Autodesk Inventor part; units mm, degrees
ref_plane "YZ Plane" through (0, 0, 0) normal (1, 0, 0) x (0, 1, 0)
ref_plane "XZ Plane" through (0, 0, 0) normal (0, 1, 0) x (-1, 0, 0)
ref_plane "XY Plane" through (0, 0, 0) normal (0, 0, 1) x (1, 0, 0)
sketch "Sketch1" plane through (0, 0, 0) normal (0, 1, 0) x (-1, 0, 0)
  line L0 (9.5, 7.5) -> (-9.5, 7.5)
  line L1 (-9.5, 7.5) -> (-9.5, -7.5)
  line L2 (-9.5, -7.5) -> (9.5, -7.5)
  line L3 (9.5, -7.5) -> (9.5, 7.5)
  line L4 (9.5, 7.5) -> (-9.5, -7.5) construction
  line L5 (-9.5, 7.5) -> (9.5, -7.5) construction
  line L6 (7.5, 5.5) -> (-7.5, 5.5)
  line L7 (-7.5, 5.5) -> (-7.5, -5.5)
  line L8 (-7.5, -5.5) -> (7.5, -5.5)
  line L9 (7.5, -5.5) -> (7.5, 5.5)
  line L10 (7.5, 5.5) -> (-7.5, -5.5) construction
  line L11 (-7.5, 5.5) -> (7.5, -5.5) construction
  point P0 (0, 0)
  dimension "d0" = 19
  dimension "d1" = 15
  dimension "d2" = 2
  dimension "d3" = 2
extrude "Extrusion1" add sketch "Sketch1" along normal blind 115
sketch "Sketch3" plane through (0, 0, 0) normal (0, -1, 0) x (1, 0, 0)
  circle A0 centre (2.5, 11.5) radius 2.5
  circle A1 centre (2.5, -11.5) radius 2.5
  line L0 (-9.5, -7.5) -> (-9.5, 7.5)
  line L1 (-9.5, 7.5) -> (9.5, 7.5)
  line L2 (-2, 7.5) -> (7, 7.5)
  line L3 (7, 7.5) -> (7, 16.5)
  line L4 (7, 16.5) -> (-2, 16.5)
  line L5 (-2, 16.5) -> (-2, 7.5)
  line L6 (0, 0) -> (7.5, 0)
  line L7 (7.5, -5.5) -> (7.5, 5.5)
  circle A2 centre (2.5, -11.5) radius 2.5
  line L8 (-9.5, -7.5) -> (9.5, -7.5)
  line L9 (7, -7.5) -> (7, -16.5)
  line L10 (7, -16.5) -> (-2, -16.5)
  line L11 (-2, -16.5) -> (-2, -7.5)
  dimension "d13" = 5
  dimension "d14" = 5
  dimension "d15" = 23
  dimension "d16" = 11.5
  dimension "d17" = 12
  dimension "d18" = 12
  dimension "d19" = 9
  dimension "d20" = 9
  dimension "d21" = 4.5
extrude "Extrusion3" add sketch "Sketch3" against normal blind 3
fillet "Fillet2" radius 2 8 edges at (-2, 1.5, -7.5) (-2, 1.5, -16.5) (7, 1.5, -16.5) (7, 1.5, -7.5) (7, 1.5, 7.5) (7, 1.5, 16.5) (-2, 1.5, 16.5) (-2, 1.5, 7.5)
sketch "Sketch2" plane through (0, 0, 0) normal (0, -1, 0) x (1, 0, 0)
  circle A0 centre (-11.5, 0) radius 2.5
  circle A1 centre (11.5, 0) radius 2.5
  line L0 (-14.8361, 4.3238) -> (-8.1639, 4.3238)
  line L1 (-8.1639, 4.3238) -> (-8.1639, -4.3238)
  line L2 (-8.1639, -4.3238) -> (-14.8361, -4.3238)
  line L3 (-14.8361, -4.3238) -> (-14.8361, 4.3238)
  line L4 (-14.8361, 4.3238) -> (-8.1639, -4.3238) construction
  line L5 (-8.1639, 4.3238) -> (-14.8361, -4.3238) construction
  line L6 (0, 0) -> (0, 5.5)
  line L7 (7.5, 5.5) -> (-7.5, 5.5)
  line L8 (14.8361, 4.3238) -> (8.1639, 4.3238)
  line L9 (8.1639, 4.3238) -> (8.1639, -4.3238)
  line L10 (8.1639, -4.3238) -> (14.8361, -4.3238)
  line L11 (14.8361, -4.3238) -> (14.8361, 4.3238)
  dimension "d6" = 5
  dimension "d7" = 5
  dimension "d8" = 23
  dimension "d9" = 11.5
properties part number "neck"
Check sheet for the modelled part. Datum: model origin and axes. Units: mm. A direction names the side the tool comes from. Round coordinates to 2 decimals unless told otherwise and drop trailing zeros. Order: outer loops, then holes, each group sorted by start corner. A loop starts at its lowest first (then second) coordinate and runs counter-clockwise, first axis right, second up.
(1) Scan lines: probe 1 along Z at (x, y) = (2.5, 1.45); probe 2 along Z at (x, y) = (-0.75, 43.5); probe 3 along X at (y, z) = (60, 0). Record each from-to range of solid material in increasing order.
(2) Cross-section at C-C, the plane x = 2.5. Enter the section's corners in (y, z).
(3) Go/stop test with flat-tipped pins: P1, Ø2.5, axis at y = 1, z = 12, coming from the -X side; P2, Ø7, axis at x = 0.5, z = -13, coming from the +Y side; P3, Ø3.5, axis at y = 1.5, z = 12, coming from the +X side. Record where each tip stops, or that it passes through.
(4) Cross-section at A-A, the plane z = 2. Enter the section's corners in (x, y), and give its area (3 significant figures).
(5) Cross-section at D-D, the plane z = -11.5. Enter the section's corners in (x, y).
(6) Access from +Z, -Z, +X, -X, +Y, -Y to the whole of each face (thin tool, end or side, straight path). Record for faces 5 (the flat face through (7, 1, -12)), 6 (the flat face through (4, 3, -14)), 7 (the cylindrical face through (-1.43, 1.52, 15.9)), 8 (the flat face through (7, 1, 12)), 9 (the flat face through (3, 1, 16.5)).
(7) Draft check along X on faces 1 (the flat face through (0, 57, 5.5)), 2 (the flat face through (-2, 1, 12)), 3 (the flat face through (3, 1, -16.5)), 4 (the flat face through (7.5, 57, 0)). Enter one of: pulls with the +X half, pulls with the -X half, needs draft (parallel to the pull), parting line crosses it, or undercut.
(8) Cross-section at B-B, the plane y = 9.5. Enter the section's corners in (x, z), and give its area (3 significant figures).
Check sheet entries:
1. probe 1: z = -16.5 to -14, -9 to -5.5, 5.5 to 9, 14 to 16.5
1. probe 2: z = -7.5 to -5.5, 5.5 to 7.5
1. probe 3: x = -9.5 to -7.5, 7.5 to 9.5
2. outline: (0, -16.5) - (3, -16.5) - (3, -14) - (0, -14) - close; (0, -9) - (3, -9) - (3, -7.5) - (115, -7.5) - (115, -5.5) - (0, -5.5) - close; (0, 5.5) - (115, 5.5) - (115, 7.5) - (3, 7.5) - (3, 9) - (0, 9) - close; (0, 14) - (3, 14) - (3, 16.5) - (0, 16.5) - close
3. P1: stops at x = -2
3. P2: stops at y = 3
3. P3: stops at x = 7
4. outline: (-9.5, 0) - (-7.5, 0) - (-7.5, 115) - (-9.5, 115) - close; (7.5, 0) - (9.5, 0) - (9.5, 115) - (7.5, 115) - close
4. area: 460 mm2
5. outline: (-2, 0) - (0, 0) - (0, 3) - (-2, 3) - close; (5, 0) - (7, 0) - (7, 3) - (5, 3) - close
6. face 5: -Z, +X, +Y, -Y
6. face 6: -Z, +X, -X, +Y
6. face 7: +Z, -X, +Y, -Y
6. face 8: +Z, +X, +Y, -Y
6. face 9: +Z, +X, -X, +Y, -Y
7. face 1: undercut
7. face 2: pulls with the -X half
7. face 3: needs draft
7. face 4: undercut
8. outline: (-9.5, -7.5) - (9.5, -7.5) - (9.5, 7.5) - (-9.5, 7.5) - close; hole (-7.5, -5.5) - (7.5, -5.5) - (7.5, 5.5) - (-7.5, 5.5) - close
8. area: 120 mm2
